Part model, mm, in its own coordinate system. Face numbers are marked on the shaded views. A direction names the side the tool comes from. Give positions to 0.01 mm unless a question says otherwise; leave off trailing zeros. Loops run counter-clockwise (first coordinate to the right, second up) from the corner with the lowest first, then second, coordinate; pieces in that order, holes last. Notation, with made-up numbers: (34, 28.5) -> (84, 28.5) arc R29 cw to (84, 57.5) -> close; hole circle Ø3 at (39.25, 37.5). An arc over 180 degrees is marked (long way). Write item = value, one per line.
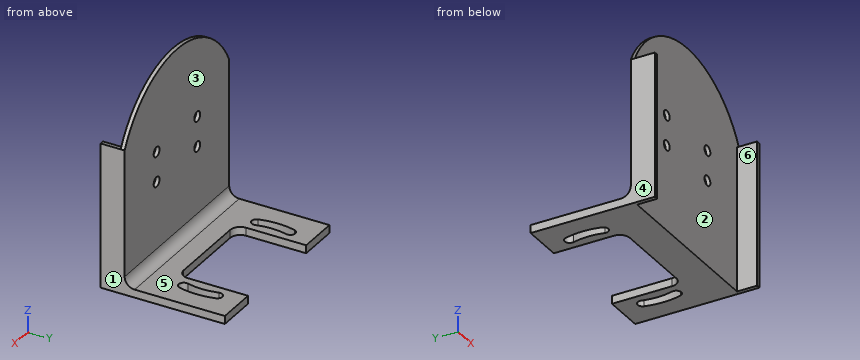
from build123d import *

# Parameters (mm, degrees)
SKETCH1_W                = 200
SKETCH1_H                = 100
BOSS_EXTRUDE1_DEPTH      = 2
BOSS_EXTRUDE2_DEPTH      = 50
CUT_EXTRUDE6_DEPTH       = 50
CUT_EXTRUDE7_DEPTH       = 50
SKETCH9_R                = 2.5
CUT_EXTRUDE8_DEPTH       = 20
CUT_EXTRUDE20_DEPTH      = 123.474487139
CUT_EXTRUDE20_DEPTH_BACK = 123.474487139
BOSS_EXTRUDE5_DEPTH      = 90
CUT_EXTRUDE28_DEPTH      = 84.815273071
CUT_EXTRUDE28_DEPTH_BACK = 84.815273071
SKETCH25_W               = 2
SKETCH25_H               = 72.093516731
BOSS_EXTRUDE7_DEPTH      = 10


with BuildPart() as part:
    # Sketch1 → Boss-Extrude1 (new body)
    with BuildSketch(Plane(origin=(0, 0, 0), x_dir=(1, 0, 0), z_dir=(0, 1, 0))):
        Rectangle(SKETCH1_W, SKETCH1_H)
    extrude(amount=BOSS_EXTRUDE1_DEPTH)

    # Sketch3 → Boss-Extrude2 (add)
    with BuildSketch(Plane(origin=(0, 2, 0), x_dir=(1, 0, 0), z_dir=(0, 1, 0))):
        Polygon((0, 50), (-45, 50), (-45, 46), (45, 46), (45, 50), align=None)
    extrude(amount=BOSS_EXTRUDE2_DEPTH)

    # Sketch4 → Cut-Extrude6 (cut)
    with BuildSketch(Plane(origin=(0, 0, -50), x_dir=(-1, 0, 0), z_dir=(0, 0, -1))):
        with BuildLine():
            Line((25, 52), (25, 22))
            ThreePointArc((25, 22), (23.535533906, 18.464466094), (20, 17))
            Line((20, 17), (-20, 17))
            ThreePointArc((-20, 17), (-23.535533906, 18.464466094), (-25, 22))
            Line((-25, 22), (-25, 52))
            Line((-25, 52), (25, 52))
        make_face()
    extrude(amount=-CUT_EXTRUDE6_DEPTH, mode=Mode.SUBTRACT)

    # Sketch5 → Cut-Extrude7 (cut)
    with BuildSketch(Plane(origin=(0, 0, -50), x_dir=(-1, 0, 0), z_dir=(0, 0, -1))):
        with BuildLine():
            ThreePointArc((-28.977774789, 39.764571353), (-30, 32), (-28.977774789, 24.235428647))
            ThreePointArc((-28.977774789, 24.235428647), (-30.745541742, 21.173566468), (-33.80740392, 22.941333421))
            ThreePointArc((-33.80740392, 22.941333421), (-35, 32), (-33.80740392, 41.058666579))
            ThreePointArc((-33.80740392, 41.058666579), (-30.745541742, 42.826433532), (-28.977774789, 39.764571353))
        make_face()
        with BuildLine():
            ThreePointArc((28.977774789, 24.235428647), (30.745541742, 21.173566468), (33.80740392, 22.941333421))
            ThreePointArc((33.80740392, 22.941333421), (35, 32), (33.80740392, 41.058666579))
            ThreePointArc((33.80740392, 41.058666579), (30.745541742, 42.826433532), (28.977774789, 39.764571353))
            ThreePointArc((28.977774789, 39.764571353), (30, 32), (28.977774789, 24.235428647))
        make_face()
    extrude(amount=-CUT_EXTRUDE7_DEPTH, mode=Mode.SUBTRACT)

    # Sketch9 → Cut-Extrude8 (cut)
    with BuildSketch(Plane(origin=(0, 2, 0), x_dir=(1, 0, 0), z_dir=(0, 1, 0))):
        with Locations(Location((-17.5, 7.5, 0), (0, 0, 270))):
            Circle(SKETCH9_R)
        with Locations(Location((17.5, 7.5, 0), (0, 0, 90))):
            Circle(SKETCH9_R)
        with Locations(Location((17.5, -7.5, 0), (0, 0, 270))):
            Circle(SKETCH9_R)
        with Locations(Location((-17.5, -7.5, 0), (0, 0, 90))):
            Circle(SKETCH9_R)
    extrude(amount=-CUT_EXTRUDE8_DEPTH, mode=Mode.SUBTRACT)

    # Sketch17 → Cut-Extrude20 (cut, two sides: drawn at the far end of the back side and taken through both)
    with BuildSketch(Plane(origin=(0, 2, 0), x_dir=(1, 0, 0), z_dir=(0, 1, 0)).offset(-CUT_EXTRUDE20_DEPTH_BACK)):
        Polygon((-45, 46), (-45, 50), (-100, 50), (-100, -50), (-45, -50), align=None)
        Polygon((45, 50), (45, 46), (45, -50), (100, -50), (100, 50), align=None)
    extrude(amount=CUT_EXTRUDE20_DEPTH + CUT_EXTRUDE20_DEPTH_BACK, mode=Mode.SUBTRACT)

    # Sketch18 → Boss-Extrude5 (add)
    with BuildSketch(Plane.ZY.offset(45)):
        with BuildLine():
            Line((-46, 7), (-46, 2))
            Line((-46, 2), (-41, 2))
            ThreePointArc((-41, 2), (-44.535533906, 3.464466094), (-46, 7))
        make_face()
    extrude(amount=-BOSS_EXTRUDE5_DEPTH)

    # Sketch24 → Cut-Extrude28 (cut, two sides: drawn at the far end of the back side and taken through both)
    with BuildSketch(Plane(origin=(0, 2, 0), x_dir=(1, 0, 0), z_dir=(0, 1, 0)).offset(-CUT_EXTRUDE28_DEPTH_BACK)):
        with BuildLine():
            Line((-151.955597575, 193.459233006), (-45, -22.093516731))
            ThreePointArc((-45, -22.093516731), (0, -50), (45, -22.093516731))
            Line((45, -22.093516731), (151.955597575, 193.459233006))
            Line((151.955597575, 193.459233006), (151.955597575, -287.79948233))
            Line((151.955597575, -287.79948233), (-151.955597575, -287.79948233))
            Line((-151.955597575, -287.79948233), (-151.955597575, 193.459233006))
        make_face()
    extrude(amount=CUT_EXTRUDE28_DEPTH + CUT_EXTRUDE28_DEPTH_BACK, mode=Mode.SUBTRACT)

    # Sketch25 → Boss-Extrude7 (add)
    with BuildSketch(Plane.XZ):
        with Locations((-44, -13.953241634)):
            Rectangle(SKETCH25_W, SKETCH25_H)
        with Locations((44, -13.953241634)):
            Rectangle(SKETCH25_W, SKETCH25_H)
    extrude(amount=BOSS_EXTRUDE7_DEPTH)


solid = part.part
1) Drop flat-ended pins along their axis: P1, Ø12, axis at x = 3, z = 19.5, coming from the +Y side; P2, Ø0.6, axis at x = -43.5, y = -6, coming from the +Z side; P3, Ø6, axis at x = 17.5, z = 7.5, coming from the -Y side. Give the stop position or say it passes through.
Resolved:
P1 = 2
P2 = 22.09
P3 = 0
2) Slice it at D-D, the plane x = 17.5. List the corners of the cut face in (y, z).
Resolved:
outline = (0, -50) -> (17, -50) -> (17, -46) -> (7, -46) arc R5 cw to (2, -41) -> (2, -10) -> (0, -10) -> close; (0, -5) -> (2, -5) -> (2, 5) -> (0, 5) -> close; (0, 10) -> (2, 10) -> (2, 46.85) -> (0, 46.85) -> close
3) Slice it at A-A, the plane y = -2. List the corners of the cut face in (x, z).
Resolved:
outline = (-45, -50) -> (-43, -50) -> (-43, 22.09) -> (-45, 22.09) -> close; (43, -50) -> (45, -50) -> (45, 22.09) -> (43, 22.09) -> close
4) Which spindle directions (+Z, -Z, +X, -X, +Y, -Y) get a long thin tool onto all of the face, cutting with end or side? Do the marked faces 4, 5 and 6. Say none if no direction does.
Resolved:
face_4 = +Z, -Z, -X, +Y, -Y
face_5 = +Z, +X, -X, +Y
face_6 = +Z, -Z, -Y
5) Slice it at B-B, the plane z = 7.5. List the corners of the cut face in (x, y), and give its area (3 significant figures).
Resolved:
outline = (-45, -10) -> (-43, -10) -> (-43, 0) -> (-20, 0) -> (-20, 2) -> (-45, 2) -> close; (-15, 0) -> (15, 0) -> (15, 2) -> (-15, 2) -> close; (20, 0) -> (43, 0) -> (43, -10) -> (45, -10) -> (45, 2) -> (20, 2) -> close
area = 200 mm²
6) Pull direction X, two halves, no side cores. Call the marked faces 1, 2 and 3: pulls with the +X half, pulls with the -X half, needs draft (parallel to the pull), parting line crosses it, or undercut.
Resolved:
face_1 = pulls with the +X half
face_2 = undercut
face_3 = needs draft
7) Drill centre lines: line 1 along X through (y, z) = (1.1, 7.5); line 2 along Z through (x, y) = (-17, 1); line 3 along X through (y, z) = (1, 7). Where is each one in solid material? Low to high. Write a range as [from, to].
Resolved:
line_1 = [-45, -20], [-15, 15], [20, 45]
line_2 = [-50, -9.95], [-5.05, 5.05], [9.95, 47.04]
line_3 = [-45, -19.95], [-15.05, 15.05], [19.95, 45]
8) Slice it at C-C, the plane z = -35.5. List the corners of the cut face in (x, y).
Resolved:
outline = (-45, -10) -> (-43, -10) -> (-43, 0) -> (43, 0) -> (43, -10) -> (45, -10) -> (45, 2) -> (-45, 2) -> close
